from build123d import *

# Parameters (mm, degrees)
SKETCH1_R           = 31.75
BOSS_EXTRUDE1_DEPTH = 9.779
SKETCH2_R           = 2.4384
CUT_EXTRUDE1_DEPTH  = 46.95382292
CIRPATTERN1_COUNT   = 6
SKETCH3_R           = 20.955
SKETCH3_R_2         = 17.8435
CUT_EXTRUDE2_DEPTH  = 2
SKETCH4_R           = 10
SKETCH4_R_2         = 8
BOSS_EXTRUDE2_DEPTH = 12.7
SKETCH5_R           = 14.986
BOSS_EXTRUDE3_DEPTH = 3.048
SKETCH6_R           = 8.763
CUT_EXTRUDE3_DEPTH  = 2.54
SKETCH8_R           = 8
CUT_EXTRUDE4_DEPTH  = 51.443306484


with BuildPart() as part:
    # Sketch1 → Boss-Extrude1 (new body)
    with BuildSketch(Plane(origin=(0, 0, 0), x_dir=(1, 0, 0), z_dir=(0, 1, 0))):
        with Locations(Location((0, 0, 0), (0, 0, 270))):
            Circle(SKETCH1_R)
    extrude(amount=BOSS_EXTRUDE1_DEPTH)

    # Sketch2 → Cut-Extrude1 (cut, through all)
    with BuildSketch(Plane(origin=(0, 9.779, 0), x_dir=(1, 0, 0), z_dir=(0, 1, 0))):
        with Locations(Location((-24.125, 0, 0), (0, 0, 270))):
            Circle(SKETCH2_R)
    cut_extrude1 = extrude(amount=-CUT_EXTRUDE1_DEPTH, mode=Mode.SUBTRACT)

    # CirPattern1: Cut-Extrude1 ×6 about axis
    cirpattern1_axis = Axis((0, 0, 0), (0, 1, 0))
    for i in range(1, CIRPATTERN1_COUNT):
        add(cut_extrude1.rotate(cirpattern1_axis, i * 360 / CIRPATTERN1_COUNT), mode=Mode.SUBTRACT)

    # Sketch3 → Cut-Extrude2 (cut)
    with BuildSketch(Plane.XZ):
        with Locations(Location((0, 0, 0), (0, 0, 270))):
            Circle(SKETCH3_R)
        with Locations(Location((0, 0, 0), (0, 0, 270))):
            Circle(SKETCH3_R_2, mode=Mode.SUBTRACT)
    extrude(amount=-CUT_EXTRUDE2_DEPTH, mode=Mode.SUBTRACT)

    # Sketch4 → Boss-Extrude2 (add)
    with BuildSketch(Plane(origin=(0, 9.779, 0), x_dir=(1, 0, 0), z_dir=(0, 1, 0))):
        with Locations(Location((0, 0, 0), (0, 0, 270))):
            Circle(SKETCH4_R)
        with Locations(Location((0, 0, 0), (0, 0, 270))):
            Circle(SKETCH4_R_2, mode=Mode.SUBTRACT)
    extrude(amount=BOSS_EXTRUDE2_DEPTH)

    # Sketch5 → Boss-Extrude3 (add)
    with BuildSketch(Plane(origin=(0, 22.479, 0), x_dir=(1, 0, 0), z_dir=(0, 1, 0))):
        with Locations(Location((0, 0, 0), (0, 0, 90))):
            Circle(SKETCH5_R)
    extrude(amount=BOSS_EXTRUDE3_DEPTH)

    # Sketch6 → Cut-Extrude3 (cut)
    with BuildSketch(Plane(origin=(0, 25.527, 0), x_dir=(1, 0, 0), z_dir=(0, 1, 0))):
        with Locations(Location((0, 0, 0), (0, 0, 270))):
            Circle(SKETCH6_R)
    extrude(amount=-CUT_EXTRUDE3_DEPTH, mode=Mode.SUBTRACT)

    # Sketch7 → Revolve1 (revolve)
    with BuildSketch(Plane.XY, mode=Mode.PRIVATE) as revolve1_sk:
        Polygon((-14.986, 22.479), (-10, 22.479), (-10, 21.143005327), align=None)
    revolve(revolve1_sk.sketch.rotate(Axis((0, 0, 0), (0, 1, 0)), 90), axis=Axis((0, 0, 0), (0, 1, 0)))

    # Sketch8 → Cut-Extrude4 (cut, through all)
    with BuildSketch(Plane(origin=(0, 22.987, 0), x_dir=(1, 0, 0), z_dir=(0, 1, 0))):
        with Locations(Location((0, 0, 0), (0, 0, 270))):
            Circle(SKETCH8_R)
    extrude(amount=-CUT_EXTRUDE4_DEPTH, mode=Mode.SUBTRACT)


solid = part.part
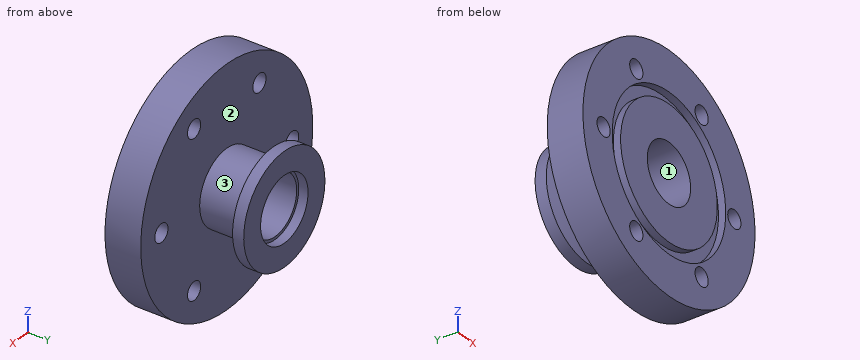
Input: part model. Units: mm. Frame: model coordinates. Face numbers are marked on the shaded views. Coordinates: 2 decimals unless noted, no trailing zeros. Write each loop counter-clockwise with the first axis right and the second up, starting at its lowest first coordinate (ties: lowest second). Pieces come first, ordered by that corner, then holes. Notation, with made-up numbers: M 39.25,-2.75 L 55.25,-2.75 A31 cw 55.25,28.25 Z; hole C 18,52 d3. An arc over 180 degrees is marked long. Answer as a JSON object with one key per item and string values. Group by question number.
(1) Mould query, pull axis Z, two halves, no side actions, for the marked faces 1, 2 and 3. Classes: pulls with the +Z half, pulls with the -Z half, needs draft (parallel to the pull), parting line crosses it, or undercut.
(2) Section C-C on y = 18.5. Output: boundary loops of the cut face in (x, z), plus the area to 3 significant figures.
(3) Section D-D on z = 26. Output: boundary loops of the cut face in (x, y).
(4) Ray query, line 1 along X through (y, z) = (2.75, 0); line 2 along X through (y, z) = (8, -2); line 3 along Y through (x, z) = (22.5, 16). Return the intervals inside material, ascending. Write a range as [from, to].
(5) Section B-B on z = 0. Give the number of separate pieces and of enclosed holes in the cut face, plus the area to 3 significant figures.
(6) Contact query for flat-ended pins moving along their axis: P1, Ø3, axis at x = 12.06, z = 20.89, coming from the -Y side; P2, Ø3, axis at x = -6, y = 16, coming from the -Z side; P3, Ø5.5, axis at x = 24.125, z = 0, coming from the -Y side; P4, Ø5, axis at y = 7, z = -22, coming from the -X side. Output: stop coordinate, or through.
Result set:
{
 "1": {"face 1": "undercut", "face 2": "needs draft", "face 3": "parting line crosses it"},
 "2": {"outline": "C 0,0 d20; hole C 0,0 d16", "area": "113 mm2"},
 "3": {"outline": "M -18.22,0 L 18.22,0 L 18.22,9.78 L -18.22,9.78 Z"},
 "4": {"line 1": "x = [-31.75, -26.56], [-21.69, -8], [8, 21.69], [26.56, 31.75]", "line 2": "x = [-31.69, -25.52], [-22.73, -7.75], [7.75, 22.73], [25.52, 31.69]", "line 3": "y = [0, 9.78]"},
 "5": {"separate pieces": "4", "enclosed holes": "0", "area": "453 mm2"},
 "6": {"P1": "passes through", "P2": "stops at z = -8.93", "P3": "stops at y = 0", "P4": "stops at x = -25.06"}
}
